```python
from build123d import *

# Parameters (mm, degrees)
SKETCH1_R               = 2.5
ALUMINIUM_PROFILE_DEPTH = 170


with BuildPart() as part:
    # Sketch1 → Aluminium_profile (new body)
    with BuildSketch(Plane.XY):
        with BuildLine():
            Line((-4.725542729, -10), (-3.125, -8.2))
            Line((-3.125, -8.2), (-5.5, -8.2))
            Line((-5.5, -8.2), (-5.5, -6.560660172))
            Line((-5.5, -6.560660172), (-2.539339828, -3.6))
            Line((-2.539339828, -3.6), (2.539339828, -3.6))
            Line((2.539339828, -3.6), (5.5, -6.560660172))
            Line((5.5, -6.560660172), (5.5, -8.2))
            Line((5.5, -8.2), (3.125, -8.2))
            Line((3.125, -8.2), (4.434457271, -10))
            Line((4.434457271, -10), (8, -10))
            ThreePointArc((8, -10), (9.414213562, -9.414213562), (10, -8))
            Line((10, -8), (10, -4.434457271))
            Line((10, -4.434457271), (8.2, -3.125))
            Line((8.2, -3.125), (8.2, -5.5))
            Line((8.2, -5.5), (6.560660172, -5.5))
            Line((6.560660172, -5.5), (3.6, -2.539339828))
            Line((3.6, -2.539339828), (3.6, 2.539339828))
            Line((3.6, 2.539339828), (6.560660172, 5.5))
            Line((6.560660172, 5.5), (8.2, 5.5))
            Line((8.2, 5.5), (8.2, 3.125))
            Line((8.2, 3.125), (10, 4.725542729))
            Line((10, 4.725542729), (10, 8))
            ThreePointArc((10, 8), (9.414213562, 9.414213562), (8, 10))
            Line((8, 10), (4.725542729, 10))
            Line((4.725542729, 10), (3.125, 8.2))
            Line((3.125, 8.2), (5.5, 8.2))
            Line((5.5, 8.2), (5.5, 6.560660172))
            Line((5.5, 6.560660172), (2.539339828, 3.6))
            Line((2.539339828, 3.6), (-2.539339828, 3.6))
            Line((-2.539339828, 3.6), (-5.5, 6.560660172))
            Line((-5.5, 6.560660172), (-5.5, 8.2))
            Line((-5.5, 8.2), (-3.125, 8.2))
            Line((-3.125, 8.2), (-4.434457271, 10))
            Line((-4.434457271, 10), (-8, 10))
            ThreePointArc((-8, 10), (-9.414213562, 9.414213562), (-10, 8))
            Line((-10, 8), (-10, 4.434457271))
            Line((-10, 4.434457271), (-8.2, 3.125))
            Line((-8.2, 3.125), (-8.2, 5.5))
            Line((-8.2, 5.5), (-6.560660172, 5.5))
            Line((-6.560660172, 5.5), (-3.6, 2.539339828))
            Line((-3.6, 2.539339828), (-3.6, -2.539339828))
            Line((-3.6, -2.539339828), (-6.560660172, -5.5))
            Line((-6.560660172, -5.5), (-8.2, -5.5))
            Line((-8.2, -5.5), (-8.2, -3.125))
            Line((-8.2, -3.125), (-10, -4.725542729))
            Line((-10, -4.725542729), (-10, -8))
            ThreePointArc((-10, -8), (-9.414213562, -9.414213562), (-8, -10))
            Line((-8, -10), (-4.725542729, -10))
        make_face()
        Circle(SKETCH1_R, mode=Mode.SUBTRACT)
    extrude(amount=ALUMINIUM_PROFILE_DEPTH)


solid = part.part
```
Read the model definition and answer for the solid it produces. Units are mm, in the model's axes. A direction names the side the tool comes from. Give positions to 0.01 mm unless a question says otherwise; leave off trailing zeros. Write each loop counter-clockwise with the first axis right and the second up, starting at its lowest first coordinate (ties: lowest second). Pieces come first, ordered by that corner, then holes. Notation, with made-up numbers: M 63.5,24 L 85.5,24 A20 cw 85.5,45 Z; hole C 84.25,-21 d6. An arc over 180 degrees is marked long. Put each result on its own line as item: value. Start each with the question number.
1. Which of the six approach directions +Z, -Z, +X, -X, +Y, -Y give full straight-line access (tool end or side, diameter ignored) to faces 1 (the flat face through (0, 3.6, 84)), 2 (the flat face through (-10, -6, 84)), 3 (the flat face through (3.6, 0, 84)), 4 (the flat face through (-3.6, 0, 84)), 5 (the flat face through (-5.1, 4.04, 83.81))?
2. For a pull along Y with two mould halves and no side action, classify faces 6 (the flat face through (0, -3.6, 84)), 7 (the flat face through (-2, 2, 170)), 8 (the flat face through (5.1, -4.04, 83.81)) as released by +Y, released by -Y, zero draft, split by the parting line, or undercut.
3. Consider line 1 along Y through (x, z) = (0, 104); line 2 along Y through (x, z) = (-5, 110.5); line 3 along X through (y, z) = (-5.25, 139.5). Determine where each line is inside the solid, lowest interval first.
4. The part is cut by section A-A, the plane x = 0. Give the vertices of the cut face in (y, z), and give its area (3 significant figures).
5. Each of these flat-tipped pins is pushed along its axis until it touches: pin 1 Ø2.5 at (x, z) = (-0.5, 89.5) entering from -Y; pin 2 Ø1.5 at (y, z) = (-0.5, 109.5) entering from +X; pin 3 Ø4 at (y, z) = (0.5, 62) entering from -X. Where does it stop, or does it pass through?
Final values:
1. face 1: +Z, -Z, +Y
1. face 2: +Z, -Z, -X, +Y, -Y
1. face 3: +Z, -Z, +X
1. face 4: +Z, -Z, -X
1. face 5: +Z, -Z
2. face 6: released by -Y
2. face 7: zero draft
2. face 8: undercut
3. line 1: y = -3.6 to -2.5, 2.5 to 3.6
3. line 2: y = -10 to -8.2, -6.06 to -3.94, 3.94 to 6.06, 8.2 to 10
3. line 3: x = -10 to -8.2, -6.31 to -4.19, 4.19 to 6.31, 8.2 to 10
4. outline: M -3.6,0 L -2.5,0 L -2.5,170 L -3.6,170 Z; M 2.5,0 L 3.6,0 L 3.6,170 L 2.5,170 Z
4. area: 374 mm²
5. pin 1: stops at y = -3.6
5. pin 2: stops at x = 3.6
5. pin 3: stops at x = -3.6
